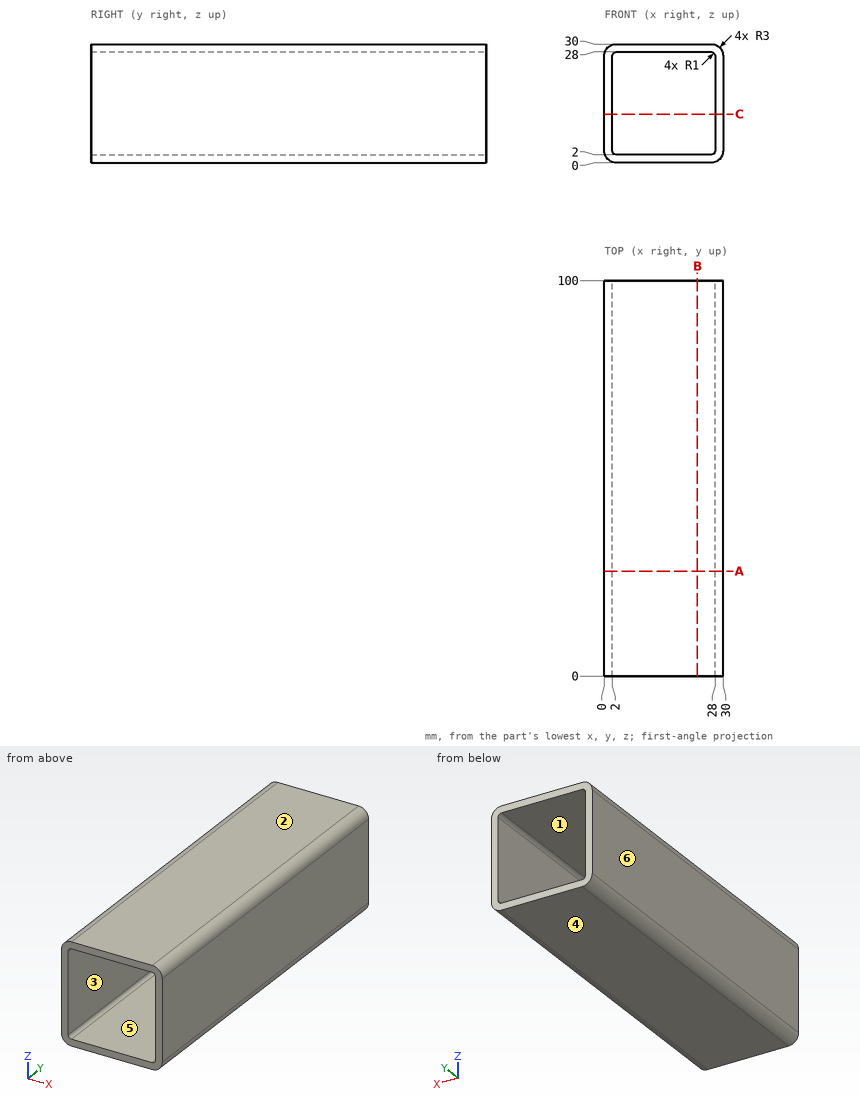
Could you check a few things on this drawing? It's one solid part, dimensions in mm from its lowest x, y, z. A direction names the side the tool comes from. Give positions to 0.01 mm unless a question says otherwise; leave off trailing zeros. Order: outer loops, then holes, each group sorted by start corner. A loop starts at its lowest first (then second) coordinate and runs counter-clockwise, first axis right, second up. Notation, with made-up numbers: (14.5, -1) - (27.5, -1) arc R15 ccw to (27.5, 6) - close; hole circle Ø9 at (-40, 59). An arc over 180 degrees is marked (long way). One line per item, written item: value. Start each with the question number.
1. For P1, Ø6, axis at x = 26, z = 11, coming from the +Y side; P2, Ø4, axis at x = 24, z = 4.5, coming from the -Y side, each with a flat end and sliding along its axis, tell me the tip position at first contact or that it passes through.
2. Imagine slicing it at C-C on z = 12.25. List the corners of the cut face in (x, y) for me.
3. Thinking about a two-plate mould opening in Z: for the marked faces 3, 4, 5 and 6, which applies, +Z half, -Z half, draft (parallel to the pull), parting line (faces both ways), or undercut?
4. Imagine slicing it at B-B on x = 23.5. List the corners of the cut face in (y, z) for me, plus the area to 3 significant figures.
5. Imagine slicing it at A-A on y = 26.5. List the corners of the cut face in (x, z) for me.
6. If I drill on probe 1 along X at (y, z) = (55, 8.75); probe 2 along Z at (x, y) = (1.5, 72.5), over which ranges is the centre line in solid material (lowest first)?
7. For the marked faces 1 and 2, which set-ups out of +Z, -Z, +X, -X, +Y, -Y let a thin tool reach every point of the face, with its end or its side?
Values:
1. P1: y = 100
1. P2: through
2. outline: (0, 0) - (2, 0) - (2, 100) - (0, 100) - close; (28, 0) - (30, 0) - (30, 100) - (28, 100) - close
3. face 3: undercut
3. face 4: -Z half
3. face 5: undercut
3. face 6: draft
4. outline: (0, 0) - (100, 0) - (100, 2) - (0, 2) - close; (0, 28) - (100, 28) - (100, 30) - (0, 30) - close
4. area: 400 mm²
5. outline: (0, 3) arc R3 ccw to (3, 0) - (27, 0) arc R3 ccw to (30, 3) - (30, 27) arc R3 ccw to (27, 30) - (3, 30) arc R3 ccw to (0, 27) - close; hole (2, 3) arc R1 ccw to (3, 2) - (27, 2) arc R1 ccw to (28, 3) - (28, 27) arc R1 ccw to (27, 28) - (3, 28) arc R1 ccw to (2, 27) - close
6. probe 1: 0 to 2, 28 to 30
6. probe 2: 0.4 to 29.6
7. face 1: +Y, -Y
7. face 2: +Z, +X, -X, +Y, -Y
